Can you work these out from the drawing? Everything is in mm from the part's minimum corner. A direction names the side the tool comes from. Give positions to 0.01 mm unless a question says otherwise; leave off trailing zeros. Loops run counter-clockwise (first coordinate to the right, second up) from the corner with the lowest first, then second, coordinate; pieces in that order, holes last. Notation, with made-up numbers: (69.5, 23) -> (76.5, 23) arc R20 cw to (76.5, 37) -> close; hole circle Ø9 at (11.25, 6). An arc over 180 degrees is marked (long way). Return JSON: item names as keys, results as strings. Group by question number.
Q1. Will these pins go through, and if not, where does the flat tip stop? pin 1 (5 mm diameter, centred on x = 43.5, y = 4, fed in from +Z); pin 2 (6 mm diameter, centred on y = 6.5, z = 31.5, fed in from -X).
Q2. Which directions (+Z, -Z, +X, -X, +Y, -Y) give clear straight access to the entire face, cutting with the end or side of a thin tool? Please do the marked faces 4 and 5.
Q3. Suppose I cut it at B-B, the plane z = 38.5. Please give me the cut outline in (x, y) (1 decimal).
Q4. Suppose I cut it at C-C, the plane x = 28. Please give me the cut outline in (y, z).
Q5. Suppose I cut it at A-A, the plane y = 4.25. Please give me the cut outline in (x, z).
Q6. Suppose I cut it at D-D, the plane y = 11.5. Please give me the cut outline in (x, z).
Q7. I need wall thicknesses on line 1 along Z through (x, y) = (39.5, 4.25) (1 decimal); line 2 along X through (y, z) = (3.5, 32) (1 decimal); line 3 along X through (y, z) = (3, 38). Which ranges of each line are inside material? Lowest first, please. Write a range as [from, to].
Q8. Thinking about a two-plate mould opening in X: for the marked faces 1, 2 and 3, which applies, pulls with the +X half, pulls with the -X half, needs draft (parallel to the pull), parting line crosses it, or undercut?
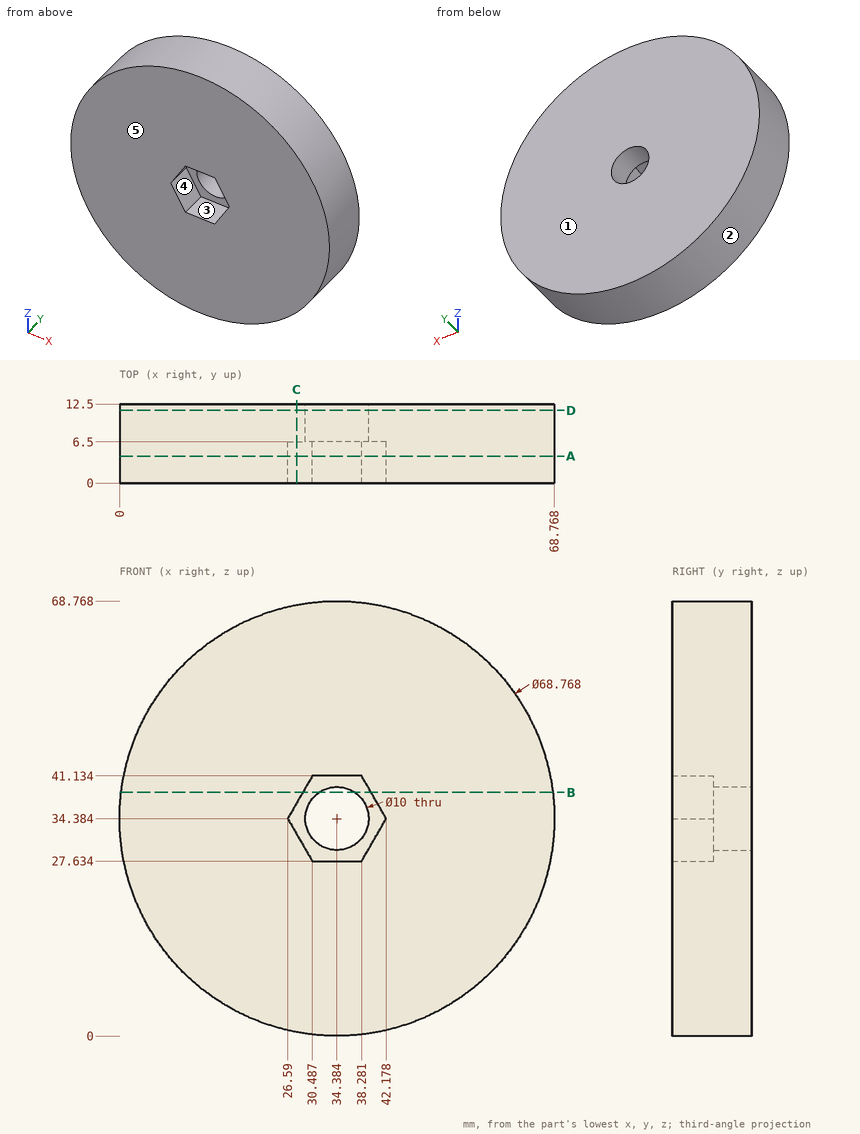
Ans:
{
 "1": {"pin 1": "stops at z = 68.13", "pin 2": "stops at x = 0"},
 "2": {"face 4": "-Y", "face 5": "+Z, -Z, +X, -X, -Y"},
 "3": {"outline": "(0.2, 0) -> (29, 0) -> (29, 6.5) -> (31.5, 6.5) -> (31.5, 12.5) -> (0.2, 12.5) -> close; (37.2, 6.5) -> (39.8, 6.5) -> (39.8, 0) -> (68.5, 0) -> (68.5, 12.5) -> (37.2, 12.5) -> close"},
 "4": {"outline": "(0, 0.6) -> (12.5, 0.6) -> (12.5, 68.17) -> (0, 68.17) -> (0, 36.83) -> (6.5, 36.83) -> (6.5, 31.94) -> (0, 31.94) -> close"},
 "5": {"outline": "circle Ø68.77 at (34.38, 34.38); hole (26.59, 34.38) -> (30.49, 27.63) -> (38.28, 27.63) -> (42.18, 34.38) -> (38.28, 41.13) -> (30.49, 41.13) -> close"},
 "6": {"outline": "circle Ø68.77 at (34.38, 34.38); hole circle Ø10 at (34.38, 34.38)"},
 "7": {"line 1": "z = [0.4, 29.7], [39, 68.4]", "line 2": "x = [0.1, 28], [40.8, 68.7]", "line 3": "x = [0.19, 28.68], [40.09, 68.58]"},
 "8": {"face 1": "needs draft", "face 2": "parting line crosses it", "face 3": "undercut"}
}
